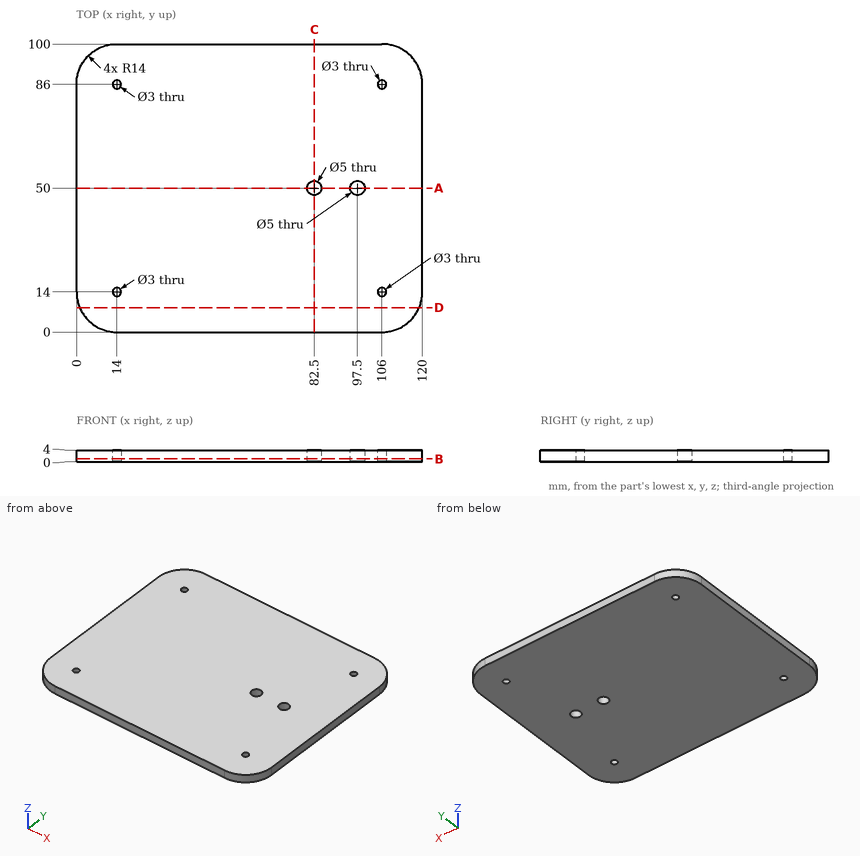
Input: dimensioned drawing with shaded views. Units: mm. Origin: part minimum x, y, z. Give positions to 0.01 mm unless a question says otherwise; leave off trailing zeros. Order: outer loops, then holes, each group sorted by start corner. A loop starts at its lowest first (then second) coordinate and runs counter-clockwise, first axis right, second up.
(1) Section query A-A (y = 50). Return the cut outline in (x, z), plus the area to 3 significant figures.
(2) Section query B-B (z = 0.95). Return the cut outline in (x, y).
(3) Contact query for a flat-ended pin moving along its axis: P1, Ø2.5, axis at x = 106, y = 86, coming from the -Z side. Output: stop coordinate, or through.
(4) Section query C-C (x = 82.5). Return the cut outline in (y, z).
(5) Section query D-D (y = 8.5). Return the cut outline in (x, z), plus the area to 3 significant figures.
(6) Material intervals for line 1 along X through (y, z) = (86, 2.7); line 2 along Y through (x, z) = (14, 2.5); line 3 along Y through (x, z) = (82.5, 2.4), sorted ascending.
Outcome:
1. outline: (0, 0) - (80, 0) - (80, 4) - (0, 4) - close; (85, 0) - (95, 0) - (95, 4) - (85, 4) - close; (100, 0) - (120, 0) - (120, 4) - (100, 4) - close
1. area: 440 mm2
2. outline: (0, 14) arc R14 ccw to (14, 0) - (106, 0) arc R14 ccw to (120, 14) - (120, 86) arc R14 ccw to (106, 100) - (14, 100) arc R14 ccw to (0, 86) - close; hole circle Ø3 at (14, 14); hole circle Ø3 at (14, 86); hole circle Ø5 at (82.5, 50); hole circle Ø5 at (97.5, 50); hole circle Ø3 at (106, 14); hole circle Ø3 at (106, 86)
3. P1: passes through
4. outline: (0, 0) - (47.5, 0) - (47.5, 4) - (0, 4) - close; (52.5, 0) - (100, 0) - (100, 4) - (52.5, 4) - close
5. outline: (1.13, 0) - (118.87, 0) - (118.87, 4) - (1.13, 4) - close
5. area: 471 mm2
6. line 1: x = 0 to 12.5, 15.5 to 104.5, 107.5 to 120
6. line 2: y = 0 to 12.5, 15.5 to 84.5, 87.5 to 100
6. line 3: y = 0 to 47.5, 52.5 to 100
